Can you work these out from the drawing? Everything is in mm from the part's minimum corner. A direction names the side the tool comes from. Round coordinates to 2 decimals unless told otherwise and drop trailing zeros. Loops run counter-clockwise (first coordinate to the right, second up) from the corner with the lowest first, then second, coordinate; pieces in that order, holes last. Notation, with made-up numbers: (6.25, 57.5) -> (21.25, 57.5) arc R21 cw to (21.25, 81.5) -> close; hole circle Ø2 at (89.5, 10). An arc over 180 degrees is marked (long way). One line per item, written item: value.
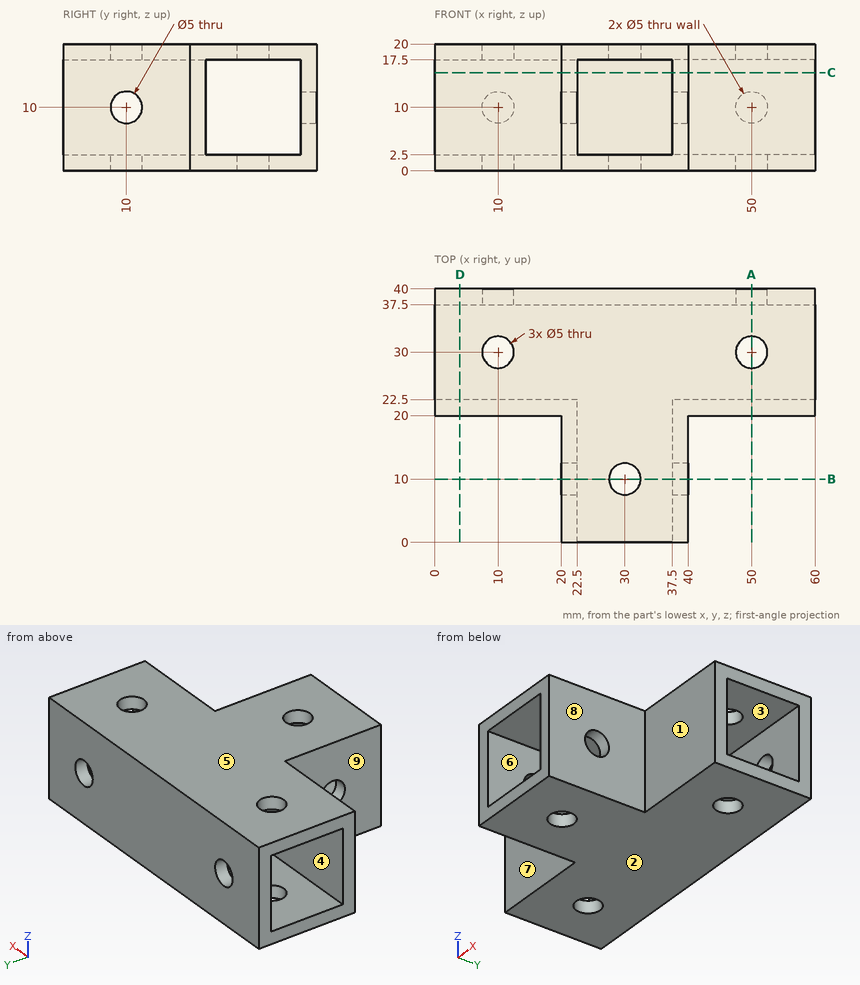
Item 1: If we section it at B-B on y = 10: List the corners of the cut face in (x, z) for me, plus the area to 3 significant figures.
Output:
outline: (20, 0) -> (27.5, 0) -> (27.5, 2.5) -> (22.5, 2.5) -> (22.5, 7.5) -> (20, 7.5) -> close; (20, 12.5) -> (22.5, 12.5) -> (22.5, 17.5) -> (27.5, 17.5) -> (27.5, 20) -> (20, 20) -> close; (32.5, 0) -> (40, 0) -> (40, 7.5) -> (37.5, 7.5) -> (37.5, 2.5) -> (32.5, 2.5) -> close; (32.5, 17.5) -> (37.5, 17.5) -> (37.5, 12.5) -> (40, 12.5) -> (40, 20) -> (32.5, 20) -> close
area: 125 mm²
Item 2: If we section it at C-C on z = 15.5: List the corners of the cut face in (x, y) for me.
Output:
outline: (0, 20) -> (20, 20) -> (20, 0) -> (22.5, 0) -> (22.5, 22.5) -> (0, 22.5) -> close; (0, 37.5) -> (60, 37.5) -> (60, 40) -> (0, 40) -> close; (37.5, 0) -> (40, 0) -> (40, 20) -> (60, 20) -> (60, 22.5) -> (37.5, 22.5) -> close
Item 3: If we section it at D-D on x = 4: List the corners of the cut face in (y, z) for me, plus the area to 3 significant figures.
Output:
outline: (20, 0) -> (40, 0) -> (40, 20) -> (20, 20) -> close; hole (22.5, 2.5) -> (37.5, 2.5) -> (37.5, 17.5) -> (22.5, 17.5) -> close
area: 175 mm²
Item 4: I need wall thicknesses on line 1 (Y direction, x = 14, z = 6.5); line 2 (Z direction, x = 10, y = 38). Which ranges of each line are inside material? Lowest first, please. Write a range as from..to.
Output:
line 1: y = 20..22.5, 37.5..40
line 2: z = 0..7.5, 12.5..20
Item 5: For the marked faces 1, 2, 3, 4 and 5, which set-ups out of +Z, -Z, +X, -X, +Y, -Y let a thin tool reach every point of the face, with its end or its side?
Output:
face 1: +Z, -Z, +X, -Y
face 2: -Z, +X, -X, +Y, -Y
face 3: none
face 4: +X, -X
face 5: +Z, +X, -X, +Y, -Y
Item 6: If we section it at A-A on x = 50: List the corners of the cut face in (y, z) for me, plus the area to 4 significant figures.
Output:
outline: (20, 0) -> (27.5, 0) -> (27.5, 2.5) -> (22.5, 2.5) -> (22.5, 17.5) -> (27.5, 17.5) -> (27.5, 20) -> (20, 20) -> close; (32.5, 0) -> (40, 0) -> (40, 7.5) -> (37.5, 7.5) -> (37.5, 2.5) -> (32.5, 2.5) -> close; (32.5, 17.5) -> (37.5, 17.5) -> (37.5, 12.5) -> (40, 12.5) -> (40, 20) -> (32.5, 20) -> close
area: 137.5 mm²
Item 7: If we mould it in two halves opening along X, with no side actions, what happens to the marked faces 6, 7, 8 and 9? For each: released by +X, released by -X, zero draft, split by the parting line, or undercut.
Output:
face 6: undercut
face 7: zero draft
face 8: released by +X
face 9: released by -X
Item 8: Will these pins go through, and if not, where does the flat tip stop? pin 1 Ø1 at (x, z) = (47, 3.5) entering from -Y; pin 2 Ø1.5 at (y, z) = (6, 9.5) entering from +X; pin 3 Ø1 at (y, z) = (30.5, 3.5) entering from +X; pin 4 Ø6 at (y, z) = (14.5, 11) entering from -X.
Output:
pin 1: stops at y = 20
pin 2: stops at x = 40
pin 3: passes through
pin 4: stops at x = 20
